The listing builds one solid part. Answer for the finished solid, in the listing's coordinates (mm). Face numbers are marked on the shaded views. A direction names the side the tool comes from. Round coordinates to 2 decimals unless told otherwise and drop trailing zeros. Write each loop counter-clockwise with the first axis right and the second up, starting at its lowest first coordinate (ties: lowest second). Pieces come first, ordered by that corner, then holes. Notation, with made-up numbers: (-35.5, 44) - (-7.5, 44) arc R22 ccw to (-7.5, 57) - close; hole circle Ø8 at (73.5, 3.5). An arc over 180 degrees is marked (long way). Use a Markdown table: item, result. Add a question column.
1) A cutting plane is placed at D-D (x = 12). Give the vertices of the cut face in (y, z).
2) Each of these flat-tipped pins is pushed along its axis until it touches: P1, Ø7.5, axis at y = -14.5, z = 7, coming from the -X side; P2, Ø4, axis at y = -14, z = -11.5, coming from the +X side; P3, Ø1.9, axis at x = -11, z = 2.5, coming from the -Y side. Where does it stop, or does it pass through?
3) A cutting plane is placed at B-B (z = -4.5). Give the vertices of the cut face in (x, y), then the cut area to 3 significant figures.
4) A cutting plane is placed at C-C (y = -2.75). Give the vertices of the cut face in (x, z).
5) Find the intervals of material crossed by probe 1 along Z at (x, y) = (12, -4.5); probe 2 along Y at (x, z) = (0, -13.9); probe 3 along X at (y, z) = (-12.5, -10.5), in increasing order. Write a range as from..to.
6) A tool of negligible diameter and unlimited length cuts with its end or side. For the marked faces 4, 5, 6, 7 and 8, from which of +Z, -Z, +X, -X, +Y, -Y can it reach the whole face along a straight path? Write none if from no direction.
7) Determine the mould class of the marked faces 1, 2 and 3 for opening direction Y: +Y half, -Y half, draft (parallel to the pull), parting line (faces both ways), or undercut.
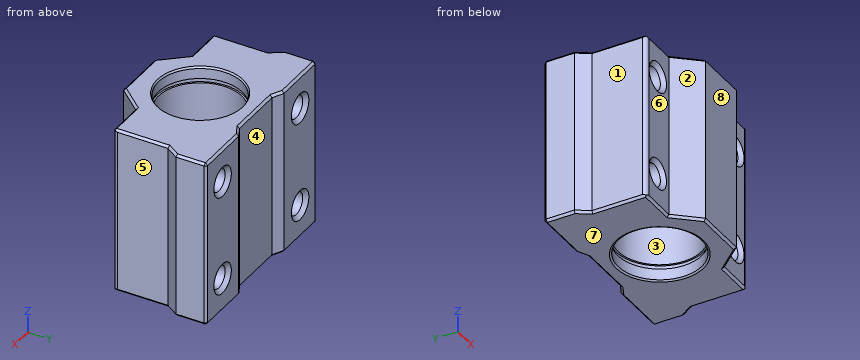
```python
from build123d import *
from OCP.BRepFilletAPI import BRepFilletAPI_MakeChamfer

# Parameters (mm, degrees)
SKETCH1_R             = 7.5
BOSS_EXTRUDE1_DEPTH   = 15
CHAFL_N0_SIZE         = 0.2
CHAFL_N0_SIZE2        = 0.346410162
CROQUIS1_R            = 2
CORTAR_EXTRUIR1_DEPTH = 20
CHAFL_N1_SIZE         = 0.7
CHAFL_N2_SIZE         = 0.4
REDONDEO1_R           = 0.7
SKETCH2_R             = 7.83
CUT_EXTRUDE1_DEPTH    = 0.8


with BuildPart() as part:
    # Sketch1 → Boss-Extrude1 (new, symmetric)
    with BuildSketch(Plane.XY):
        Polygon((-5, -1), (5, -1), (7, 0), (17, 0), (17, -5.5), (15.5, -7.8), (15.5, -17.6), (8.6, -17.6), (4.75, -22), (-4.75, -22), (-8.6, -17.6), (-15.5, -17.6), (-15.5, -7.8), (-17, -5.5), (-17, 0), (-7, 0), align=None)
        with Locations((0, -11)):
            Circle(SKETCH1_R, mode=Mode.SUBTRACT)
    extrude(amount=BOSS_EXTRUDE1_DEPTH, both=True)

    # Chaflàn0: one chamfer whose edges measure the first distance from different faces: ONE call of the kernel's chamfer builder (chamfer() names one face for all edges)
    chafl_n0_edges_1 = [part.edges().sort_by_distance(p)[0] for p in [
        (-7.5, -11, -15),
    ]]
    chafl_n0_side_1 = [part.faces().sort_by_distance(p)[0] for p in [
        (-7.5, -11, 0),
    ]]
    chafl_n0_edges_2 = [part.edges().sort_by_distance(p)[0] for p in [
        (-7.5, -11, 15),
    ]]
    chafl_n0_side_2 = [part.faces().sort_by_distance(p)[0] for p in [
        (0, -1.404969135, 15),
    ]]
    chafl_n0 = BRepFilletAPI_MakeChamfer(part.part.solid().wrapped)
    for e in chafl_n0_edges_1:
        chafl_n0.Add(CHAFL_N0_SIZE, CHAFL_N0_SIZE2, e.wrapped, chafl_n0_side_1[0].wrapped)  # the first distance lies on this face
    for e in chafl_n0_edges_2:
        chafl_n0.Add(CHAFL_N0_SIZE, CHAFL_N0_SIZE2, e.wrapped, chafl_n0_side_2[0].wrapped)  # the first distance lies on this face
    add(Compound.cast(chafl_n0.Shape()), mode=Mode.REPLACE)

    # Croquis1 → Cortar-Extruir1 (cut)
    with BuildSketch(Plane(origin=(0, 0, 0), x_dir=(1, 0, 0), z_dir=(0, 1, 0))):
        with Locations(Location((-12, 9, 0), (0, 0, 180))):
            Circle(CROQUIS1_R)
        with Locations(Location((12, 9, 0), (0, 0, 180))):
            Circle(CROQUIS1_R)
        with Locations(Location((-12, -9, 0), (0, 0, 180))):
            Circle(CROQUIS1_R)
        with Locations(Location((12, -9, 0), (0, 0, 180))):
            Circle(CROQUIS1_R)
    extrude(amount=-CORTAR_EXTRUIR1_DEPTH, mode=Mode.SUBTRACT)

    # Chaflán1
    chafl_n1_edges = [part.edges().sort_by_distance(p)[0] for p in [
        (-10, -17.6, -9),
        (-10, 0, -9),
        (14, -17.6, -9),
        (14, 0, -9),
        (-10, -17.6, 9),
        (-10, 0, 9),
        (14, -17.6, 9),
        (14, 0, 9),
    ]]
    chamfer(chafl_n1_edges, length=CHAFL_N1_SIZE)

    # Chaflán2
    chafl_n2_edges = [part.edges().sort_by_distance(p)[0] for p in [
        (-6, -0.5, 15),
        (-12, 0, 15),
        (12, 0, -15),
        (17, -2.75, -15),
        (16.25, -6.65, -15),
        (15.5, -12.7, -15),
        (12.05, -17.6, -15),
        (-17, -2.75, 15),
        (6.675, -19.8, -15),
        (0, -22, -15),
        (-6.675, -19.8, -15),
        (-12.05, -17.6, -15),
        (-15.5, -12.7, -15),
        (-16.25, -6.65, -15),
        (-17, -2.75, -15),
        (-12, 0, -15),
        (-16.25, -6.65, 15),
        (-6, -0.5, -15),
        (0, -1, -15),
        (6, -0.5, -15),
        (-15.5, -12.7, 15),
        (-12.05, -17.6, 15),
        (17, 0, 0),
        (-17, 0, 0),
        (-6.675, -19.8, 15),
        (0, -22, 15),
        (6.675, -19.8, 15),
        (12.05, -17.6, 15),
        (6, -0.5, 15),
        (15.5, -12.7, 15),
        (16.25, -6.65, 15),
        (17, -2.75, 15),
        (12, 0, 15),
        (0, -1, 15),
    ]]
    chamfer(chafl_n2_edges, length=CHAFL_N2_SIZE)

    # Redondeo1
    redondeo1_edges = [part.edges().sort_by_distance(p)[0] for p in [
        (15.5, -17.6, 0),
        (-15.5, -17.6, 0),
    ]]
    fillet(redondeo1_edges, radius=REDONDEO1_R)

    # Sketch2 → Cut-Extrude1 (cut)
    with BuildSketch(Plane.XY.offset(12.8)):
        with Locations((0, -11)):
            Circle(SKETCH2_R)
    cut_extrude1 = extrude(amount=-CUT_EXTRUDE1_DEPTH, mode=Mode.SUBTRACT)

    # Mirror1: Cut-Extrude1 across plane
    add(cut_extrude1.mirror(Plane.XY), mode=Mode.SUBTRACT)


solid = part.part
```
Entries:
| question | item | result |
|---|---|---|
| 1 | outline | (-17.6, -14.6) - (-17.2, -15) - (-0.4, -15) - (0, -14.6) - (0, -11.7) - (-0.7, -11) - (-16.9, -11) - (-17.6, -11.7) - close; (-17.6, -6.3) - (-16.9, -7) - (-0.7, -7) - (0, -6.3) - (0, 6.3) - (-0.7, 7) - (-16.9, 7) - (-17.6, 6.3) - close; (-17.6, 11.7) - (-16.9, 11) - (-0.7, 11) - (0, 11.7) - (0, 14.6) - (-0.4, 15) - (-17.2, 15) - (-17.6, 14.6) - close |
| 2 | P1 | stops at x = -15.5 |
| 2 | P2 | stops at x = 15.5 |
| 2 | P3 | stops at y = -17.6 |
| 3 | outline | (-17, -5.5) - (-15.5, -7.8) - (-15.5, -16.9) arc R0.7 ccw to (-14.8, -17.6) - (-8.6, -17.6) - (-4.75, -22) - (4.75, -22) - (8.6, -17.6) - (14.8, -17.6) arc R0.7 ccw to (15.5, -16.9) - (15.5, -7.8) - (17, -5.5) - (17, -0.4) - (16.6, 0) - (7, 0) - (5, -1) - (-5, -1) - (-7, 0) - (-16.6, 0) - (-17, -0.4) - close; hole circle Ø15 at (0, -11) |
| 3 | area | 435 mm² |
| 4 | outline | (-17, -14.6) - (-16.6, -15) - (16.6, -15) - (17, -14.6) - (17, 14.6) - (16.6, 15) - (-16.6, 15) - (-17, 14.6) - close; hole circle Ø4 at (-12, -9); hole circle Ø4 at (-12, 9); hole circle Ø4 at (12, -9); hole circle Ø4 at (12, 9) |
| 5 | probe 1 | z = -15..-11, -7..7, 11..15 |
| 5 | probe 2 | y = -22..-18.5, -3.5..-1 |
| 5 | probe 3 | x = -15.5..-13.32, -10.68..-7.35, 7.35..10.68, 13.32..15.5 |
| 6 | face 4 | +Z, -Z, +Y |
| 6 | face 5 | +Z, -Z, +X, -Y |
| 6 | face 6 | +Z, -Z, -X, -Y |
| 6 | face 7 | -Z, +X, -X, +Y, -Y |
| 6 | face 8 | +Z, -Z, +X, -X, -Y |
| 7 | face 1 | draft |
| 7 | face 2 | -Y half |
| 7 | face 3 | undercut |
